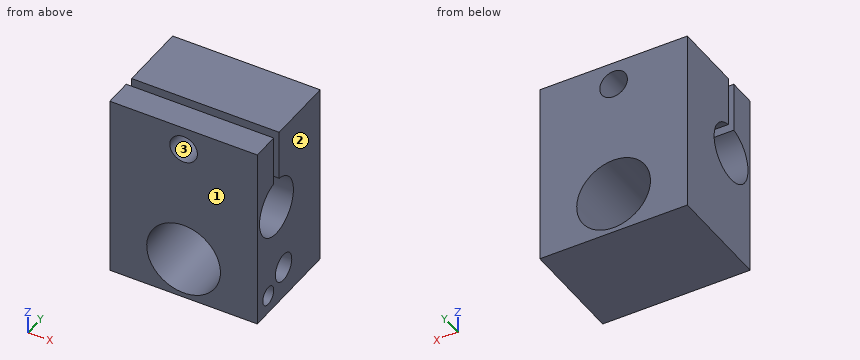
```python
from build123d import *

# Parameters (mm, degrees)
SKETCH_1_W          = 20
SKETCH_1_H          = 11.5
EXTRUDE_1_DEPTH     = 16
SKETCH_2_R          = 1.5
SKETCH_2_R_2        = 4
CUT_EXTRUDE_1_DEPTH = 29.075790283
SKETCH_6_R          = 1
CUT_EXTRUDE_2_DEPTH = 2
SKETCH_6_3_R        = 1.5
CUT_EXTRUDE_3_DEPTH = 3.8
SKETCH_6_4_R        = 3.1
CUT_EXTRUDE_4_DEPTH = 29.075790283


with BuildPart() as part:
    # Sketch 1 → Extrude 1 (new body)
    with BuildSketch(Plane(origin=(0, 0, 0), x_dir=(0, 0, -1), z_dir=(1, 0, 0))):
        with Locations((10, 5.75)):
            Rectangle(SKETCH_1_W, SKETCH_1_H)
    extrude(amount=EXTRUDE_1_DEPTH)

    # Sketch 2 → Cut-Extrude 1 (cut, through all)
    with BuildSketch(Plane(origin=(0, 11.5, 0), x_dir=(1, 0, 0), z_dir=(0, 1, 0))):
        with Locations(Location((8, 2.5, 0), (0, 0, 270))):
            Circle(SKETCH_2_R)
        with Locations(Location((8, 15.5, 0), (0, 0, 270))):
            Circle(SKETCH_2_R_2)
    extrude(amount=-CUT_EXTRUDE_1_DEPTH, mode=Mode.SUBTRACT)

    # Sketch 6 → Cut-Extrude 2 (cut)
    with BuildSketch(Plane(origin=(16, 0, 0), x_dir=(0, 0, -1), z_dir=(1, 0, 0))):
        with Locations((18, 2)):
            Circle(SKETCH_6_R)
    extrude(amount=-CUT_EXTRUDE_2_DEPTH, mode=Mode.SUBTRACT)

    # Sketch 6_3 → Cut-Extrude 3 (cut)
    with BuildSketch(Plane(origin=(16, 0, 0), x_dir=(0, 0, -1), z_dir=(1, 0, 0))):
        with Locations((16.5, 4.8)):
            Circle(SKETCH_6_3_R)
    extrude(amount=-CUT_EXTRUDE_3_DEPTH, mode=Mode.SUBTRACT)

    # Sketch 6_4 → Cut-Extrude 4 (cut, through all)
    with BuildSketch(Plane(origin=(16, 0, 0), x_dir=(0, 0, -1), z_dir=(1, 0, 0))):
        with Locations((8.5, 3.5)):
            Circle(SKETCH_6_4_R)
        with BuildLine():
            ThreePointArc((5.4, 3.5), (5.410163734, 3.750822352), (5.440588292, 4))
            Line((5.440588292, 4), (0, 4))
            Line((0, 4), (0, 3.5))
            Line((0, 3.5), (5.4, 3.5))
        make_face()
        with BuildLine():
            ThreePointArc((5.440588292, 3), (5.410163734, 3.249177648), (5.4, 3.5))
            Line((5.4, 3.5), (0, 3.5))
            Line((0, 3.5), (0, 3))
            Line((0, 3), (5.440588292, 3))
        make_face()
        with BuildLine():
            Line((8.5, 3), (8.5, 3.5))
            Line((8.5, 3.5), (5.4, 3.5))
            ThreePointArc((5.4, 3.5), (5.410163734, 3.249177648), (5.440588292, 3))
            Line((5.440588292, 3), (8.5, 3))
        make_face()
        with BuildLine():
            Line((8.5, 3.5), (8.5, 4))
            Line((8.5, 4), (5.440588292, 4))
            ThreePointArc((5.440588292, 4), (5.410163734, 3.750822352), (5.4, 3.5))
            Line((5.4, 3.5), (8.5, 3.5))
        make_face()
    extrude(amount=-CUT_EXTRUDE_4_DEPTH, mode=Mode.SUBTRACT)


solid = part.part
```
Can you work these out from the model? Positions are in its coordinate system, mm. Face numbers are marked on the shaded views. Round coordinates to 2 decimals unless told otherwise and drop trailing zeros. Loops run counter-clockwise (first coordinate to the right, second up) from the corner with the lowest first, then second, coordinate; pieces in that order, holes last. Notation, with made-up numbers: M 8.25,31.25 L 47.25,31.25 A23 ccw 47.25,54.25 Z; hole C 59.5,-34 d2. An arc over 180 degrees is marked long. Answer in a Markdown table with one row per item.
1. If we section it at C-C, the plane z = -2.5: Please give me the cut outline in (x, y), plus the area to 4 significant figures.
Established:
| item | result |
|---|---|
| outline | M 0,0 L 6.5,0 L 6.5,3 L 0,3 Z; M 0,4 L 6.5,4 L 6.5,11.5 L 0,11.5 Z; M 9.5,0 L 16,0 L 16,3 L 9.5,3 Z; M 9.5,4 L 16,4 L 16,11.5 L 9.5,11.5 Z |
| area | 136.5 mm² |
2. If we section it at A-A, the plane y = 4.8: Please give me the cut outline in (x, z).
Established:
| item | result |
|---|---|
| outline | M 0,-20 L 16,-20 L 16,-18 L 12.2,-18 L 12.2,-15 L 16,-15 L 16,-11.31 L 0,-11.31 Z; M 0,-5.69 L 16,-5.69 L 16,0 L 0,0 Z; hole C 8,-15.5 d8; hole C 8,-2.5 d3 |
3. Please list where these lines run through material, in increasing order: line 1 (X direction, y = 2, z = -2.5); line 2 (Y direction, x = 11.25, z = -4.25); line 3 (Z direction, x = 7.5, y = 1.25). Write a range as from..to.
Established:
| item | result |
|---|---|
| line 1 | 0..6.5, 9.5..16 |
| line 2 | 0..3, 4..11.5 |
| line 3 | -20..-19.47, -11.53..-10.63, -6.37..-3.91, -1.09..0 |
4. If we section it at D-D, the plane x = 13.75: Please give me the cut outline in (y, z), plus the area to 3 significant figures.
Established:
| item | result |
|---|---|
| outline | M 0,-20 L 11.5,-20 L 11.5,0 L 4,0 L 4,-5.44 A3.1 cw long 3,-5.44 L 3,0 L 0,0 Z; hole C 4.8,-16.5 d3 |
| area | 187 mm² |
5. Thinking about a two-plate mould opening in X: for the marked faces 1, 2 and 3, which applies, pulls with the +X half, pulls with the -X half, needs draft (parallel to the pull), parting line crosses it, or undercut?
Established:
| item | result |
|---|---|
| face 1 | needs draft |
| face 2 | pulls with the +X half |
| face 3 | undercut |
6. If we section it at B-B, the plane z = -8.5: Please give me the cut outline in (x, y), plus the area to 3 significant figures.
Established:
| item | result |
|---|---|
| outline | M 0,0 L 16,0 L 16,0.4 L 0,0.4 Z; M 0,6.6 L 16,6.6 L 16,11.5 L 0,11.5 Z |
| area | 84.8 mm² |
7. I'm going to push flat-ended pins straight in: pin 1 Ø1 at (y, z) = (2, -18) entering from +X; pin 2 Ø3 at (x, y) = (13.5, 8) entering from +Z. Where does each tip first touch, or does it pass through?
Established:
| item | result |
|---|---|
| pin 1 | x = 14 |
| pin 2 | z = 0 |
